```python
from build123d import *

# Parameters (mm, degrees)
BOSS_EXTRU_1_DEPTH = 5


with BuildPart() as part:
    # Esquisse1 → Boss.-Extru.1 (new body)
    with BuildSketch(Plane.XY):
        Polygon((-70, 190), (-72, 190), (-72, 185), (-84, 185), (-84, 180), (-82, 180), (-82, 181.5), (-77, 181.5), (-77, 180), (-72, 180), (-72, 170), (-77, 170), (-77, 168.5), (-82, 168.5), (-82, 170), (-84, 170), (-84, 165), (-72, 165), (-72, 145), (-77, 145), (-77, 140), (-72, 140), (-72, 130), (-77, 130), (-77, 125), (-72, 125), (-72, 105), (-77, 105), (-77, 100), (-72, 100), (-72, 90), (-77, 90), (-77, 85), (-72, 85), (-72, 65), (-77, 65), (-77, 60), (-72, 60), (-72, 50), (-77, 50), (-77, 45), (-72, 45), (-72, 25), (-77, 25), (-77, 20), (-72, 20), (-72, 10), (-77, 10), (-77, 5), (-72, 5), (-72, 0), (-70, 0), (-70, -5), (-65, -5), (-65, 0), (-55, 0), (-55, -5), (-50, -5), (-50, 0), (-30, 0), (-30, -5), (-25, -5), (-25, 0), (-15, 0), (-15, -5), (-10, -5), (-10, 0), (10, 0), (10, -5), (15, -5), (15, 0), (25, 0), (25, -5), (30, -5), (30, 0), (50, 0), (50, -5), (55, -5), (55, 0), (65, 0), (65, -5), (70, -5), (70, 0), (72, 0), (72, 5), (77, 5), (77, 10), (72, 10), (72, 20), (77, 20), (77, 25), (72, 25), (72, 45), (77, 45), (77, 50), (72, 50), (72, 60), (77, 60), (77, 65), (72, 65), (72, 85), (77, 85), (77, 90), (72, 90), (72, 100), (77, 100), (77, 105), (72, 105), (72, 125), (77, 125), (77, 130), (72, 130), (72, 140), (77, 140), (77, 145), (72, 145), (72, 165), (84, 165), (84, 170), (82, 170), (82, 168.5), (77, 168.5), (77, 170), (72, 170), (72, 180), (77, 180), (77, 181.5), (82, 181.5), (82, 180), (84, 180), (84, 185), (72, 185), (72, 190), (70, 190), (70, 195), (65, 195), (65, 190), (55, 190), (55, 195), (50, 195), (50, 190), (30, 190), (30, 195), (25, 195), (25, 190), (15, 190), (15, 195), (10, 195), (10, 190), (-10, 190), (-10, 195), (-15, 195), (-15, 190), (-25, 190), (-25, 195), (-30, 195), (-30, 190), (-50, 190), (-50, 195), (-55, 195), (-55, 190), (-65, 190), (-65, 195), (-70, 195), align=None)
        with BuildLine():
            ThreePointArc((20, 40), (0, 20), (-20, 40))
            Line((-20, 40), (-20, 70))
            ThreePointArc((-20, 70), (0, 90), (20, 70))
            Line((20, 70), (20, 40))
        make_face(mode=Mode.SUBTRACT)
        with BuildLine():
            ThreePointArc((20, 120), (0, 100), (-20, 120))
            Line((-20, 120), (-20, 150))
            ThreePointArc((-20, 150), (0, 170), (20, 150))
            Line((20, 150), (20, 120))
        make_face(mode=Mode.SUBTRACT)
    extrude(amount=BOSS_EXTRU_1_DEPTH)


solid = part.part
```
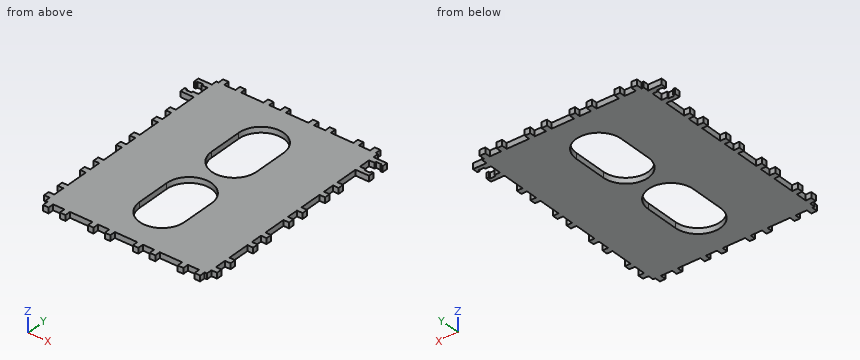
Verification items for the finished model (mm, model axes). Give positions to 0.01 mm unless a question says otherwise; leave off trailing zeros. Loops run counter-clockwise (first coordinate to the right, second up) from the corner with the lowest first, then second, coordinate; pieces in that order, holes last. Notation, with made-up numbers: M -14,36.5 L 40,36.5 A30 cw 40,59.5 Z; hole C 86,-5 d7. An arc over 180 degrees is marked long. Return JSON: item names as keys, results as strings.
1) Section check C-C, the plane y = 159. Enter the section's corners in (x, z).
Findings:
{"outline": "M -72,0 L -17.86,0 L -17.86,5 L -72,5 Z; M 17.86,0 L 72,0 L 72,5 L 17.86,5 Z"}
2) Section check B-B, the plane x = 0. Enter the section's corners in (y, z).
Findings:
{"outline": "M 0,0 L 20,0 L 20,5 L 0,5 Z; M 90,0 L 100,0 L 100,5 L 90,5 Z; M 170,0 L 190,0 L 190,5 L 170,5 Z"}
3) Section check A-A, the plane y = 134. Enter the section's corners in (x, z).
Findings:
{"outline": "M -72,0 L -20,0 L -20,5 L -72,5 Z; M 20,0 L 72,0 L 72,5 L 20,5 Z"}
4) Section check D-D, the plane z = 1.25. Count the separate pieces of the cut face and the enclosed holes in it, and give its area (3 significant figures).
Findings:
{"separate pieces": "1", "enclosed holes": "2", "area": "23,500 mm2"}
5) Material ranges on L1, parallel to Y at x = 9, z = 4.65; L2, parallel to X at y = 136.5, z = 4.8; L3, parallel to X at y = 47.5, z = 1.8, recorded low to high. Write a range as [from, to].
Findings:
{"L1": "y = [0, 22.14], [87.86, 102.14], [167.86, 190]", "L2": "x = [-72, -20], [20, 72]", "L3": "x = [-77, -20], [20, 77]"}
6) Gauge pin test, flat ends, axial feed: P1, Ø1.5, axis at y = 89, z = 2, coming from the +X side; P2, Ø1, axis at x = 71, z = 2.5, coming from the -Y side; P3, Ø1.5, axis at y = -2.5, z = 1.5, coming from the -X side. Record the tip position at first contact, or that the pin passes through.
Findings:
{"P1": "stops at x = 77", "P2": "stops at y = 0", "P3": "stops at x = -70"}
